Design review of the part built by this model. Coordinates are the model's own, in mm. Face numbers are marked on the shaded views. A direction names the side the tool comes from. Give positions to 0.01 mm unless a question says otherwise; leave off trailing zeros. Order: outer loops, then holes, each group sorted by start corner. A loop starts at its lowest first (then second) coordinate and runs counter-clockwise, first axis right, second up. Notation, with made-up numbers: M 38.25,76.5 L 54.25,76.5 A13 cw 54.25,92.5 Z; hole C 39,15 d7. An arc over 180 degrees is marked long. Answer as a JSON object with one key per item and string values.
from build123d import *

# Parameters (mm, degrees)
BOSS_EXTRUDE2_DEPTH      = 20
SKETCH8_W                = 9
SKETCH8_H                = 14
CUT_EXTRUDE1_DEPTH       = 10
CUT_EXTRUDE1_TAPER       = 1
BOSS_EXTRUDE3_START      = -10
SKETCH9_W                = 225.34
SKETCH9_H                = 10
BOSS_EXTRUDE3_DEPTH      = 20
BOSS_EXTRUDE3_DEPTH_BACK = 20


with BuildPart() as part:
    # Sketch7 → Boss-Extrude2 (new body)
    with BuildSketch(Plane.XY):
        with BuildLine():
            Line((0, 10), (0, 60))
            Line((0, 60), (15, 60))
            ThreePointArc((15, 60), (60.085, 14.915), (105.17, 60))
            Line((105.17, 60), (120.17, 60))
            ThreePointArc((120.17, 60), (165.255, 14.915), (210.34, 60))
            Line((210.34, 60), (225.34, 60))
            Line((225.34, 60), (225.34, 0))
            Line((225.34, 0), (0, 0))
            Line((0, 0), (0, 10))
        make_face()
    extrude(amount=BOSS_EXTRUDE2_DEPTH)

    # Sketch8 → Cut-Extrude1 (cut)
    with BuildSketch(Plane(origin=(0, 60, 0), x_dir=(1, 0, 0), z_dir=(0, 1, 0))):
        with Locations((7.5, -10)):
            Rectangle(SKETCH8_W, SKETCH8_H)
        with Locations((217.84, -10)):
            Rectangle(SKETCH8_W, SKETCH8_H)
        with Locations((112.67, -10)):
            Rectangle(SKETCH8_W, SKETCH8_H)
    extrude(amount=-CUT_EXTRUDE1_DEPTH, taper=CUT_EXTRUDE1_TAPER, mode=Mode.SUBTRACT)

    # Sketch9 → Boss-Extrude3 (add, two sides)
    with BuildSketch(Plane.XY.offset(20).offset(BOSS_EXTRUDE3_START)) as boss_extrude3_sk:
        with Locations((112.67, 5)):
            Rectangle(SKETCH9_W, SKETCH9_H)
    extrude(amount=BOSS_EXTRUDE3_DEPTH)
    extrude(boss_extrude3_sk.sketch, amount=-BOSS_EXTRUDE3_DEPTH_BACK)


solid = part.part
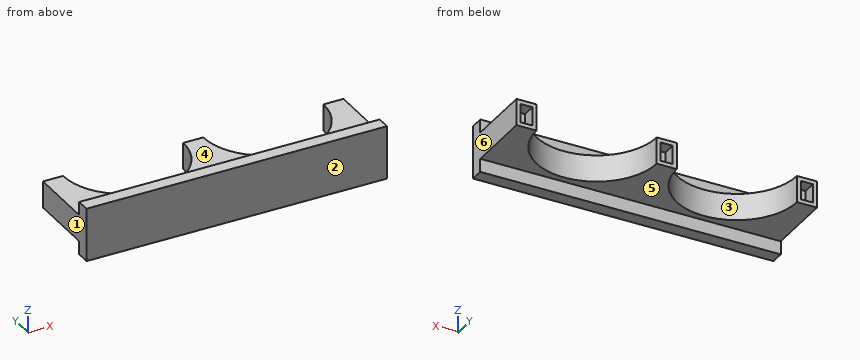
(1) Draft analysis for pull direction X (two halves, no side actions). For the marked faces 1, 2 and 3, state which applies: +X half, -X half, draft (parallel to the pull), parting line (faces both ways), or undercut.
Checked values:
{"face 1": "-X half", "face 2": "draft", "face 3": "undercut"}
(2) Insertion check: pin 1 (11 mm diameter, centred on x = 62, z = -7, fed in from +Y); pin 2 (2.5 mm diameter, centred on x = 219, z = 12, fed in from +Y); pin 3 (1 mm diameter, centred on x = 130, y = 18.5, fed in from -Z). Each pin has a flat end and moves straight along its axis. Give the tip position at first contact, or say it passes through.
Checked values:
{"pin 1": "stops at y = 10", "pin 2": "stops at y = 50", "pin 3": "stops at z = 0"}
(3) To check wall thickness, follow L1, parallel to X at y = 36, z = 18.5; L2, parallel to X at y = 39.5, z = 4; L3, parallel to X at y = 52.5, z = 4. State the ranges of each line that lie inside material, in increasing order. Write a range as from..to.
Checked values:
{"L1": "x = 0..21.92, 98.25..127.09, 203.42..225.34", "L2": "x = 0..19.93, 100.24..125.1, 205.41..225.34", "L3": "x = 0..3.13, 11.87..15.63, 104.54..108.3, 117.04..120.8, 209.71..213.47, 222.21..225.34"}
(4) We need section D-D (z = 26.5). Write out the cut boundary in (x, y), plus the area to 3 significant figures.
Checked values:
{"outline": "M 0,0 L 225.34,0 L 225.34,10 L 0,10 Z", "area": "2,250 mm^2"}
(5) We need section A-A (y = 43). Write out the cut boundary in (x, z).
Checked values:
{"outline": "M 0,0 L 18.33,0 L 18.33,20 L 0,20 Z; M 101.84,0 L 123.5,0 L 123.5,20 L 101.84,20 Z; M 207.01,0 L 225.34,0 L 225.34,20 L 207.01,20 Z"}
(6) Tool access review of the marked faces 4, 5 and 6: name each direction out of +Z, -Z, +X, -X, +Y, -Y from which nothing blocks a thin tool from reaching the whole face with its end or side.
Checked values:
{"face 4": "+Z, +X, -X, +Y", "face 5": "-Z, +X, -X, +Y", "face 6": "+Z, -Z, +X, +Y, -Y"}
(7) We need section B-B (x = 184). Write out the cut boundary in (y, z), plus the area to 3 significant figures.
Checked values:
{"outline": "M 0,-10 L 10,-10 L 10,0 L 19,0 L 19,20 L 10,20 L 10,30 L 0,30 Z", "area": "580 mm^2"}
(8) We need section C-C (y = 55). Count the separate pieces of the cut face and the enclosed holes in it, plus the area to 3 significant figures.
Checked values:
{"separate pieces": "3", "enclosed holes": "3", "area": "556 mm^2"}
